Check sheet for the modelled part. Datum: model origin and axes. Units: mm. A direction names the side the tool comes from. Coordinates: 2 decimals unless noted, no trailing zeros. Loops run counter-clockwise (first coordinate to the right, second up) from the corner with the lowest first, then second, coordinate; pieces in that order, holes last. Notation, with made-up numbers: (40.25, 75.5) - (97.25, 75.5) arc R10 cw to (97.25, 81.5) - close; hole circle Ø10 at (48.5, 21.5). An arc over 180 degrees is marked (long way). Use a Markdown table: item, result. Add a question column.
1) Sectioned sample at B-B, the plane y = 0. Enter the section's corners in (x, z), then the cut area to 4 significant figures.
2) Draft check along Y on faces 1 (the flat face through (0, 0, 17)), 2 (the flat face through (0, 2, 10.5)), 3 (the cylindrical face through (-2.17, -9.76, 8.38)). Enter one of: pulls with the +Y half, pulls with the -Y half, needs draft (parallel to the pull), parting line crosses it, or undercut.
3) Go/stop test with flat-tipped pins: P1, Ø1.3, axis at x = 1, y = 1, coming from the -Z side; P2, Ø10, axis at y = 7, z = 13, coming from the +X side; P3, Ø2, axis at y = -6.5, z = 11.5, coming from the +X side; P4, Ø8, axis at y = -3.5, z = 8, coming from the -X side. Record where each tip stops, or that it passes through.
4) Sectioned sample at A-A, the plane x = 0. Enter the section's corners in (y, z).
5) Sectioned sample at D-D, the plane z = 2.25. Enter the section's corners in (x, y), then the cut area to 3 significant figures.
6) Thickness scan on line 1 (Y direction, x = 0, z = 2.1); line 2 (Z direction, x = 5, y = -1.25); line 3 (X direction, y = 6.25, z = 2.5). Record the ranges inside material, lowest first.
7) Sectioned sample at C-C, the plane z = 8. Enter the section's corners in (x, y), then the cut area to 3 significant figures.
8) Tool access check on faces 4 (the flat face through (4, 7, 0)), 5 (the flat face through (0, 0, 3.5)). Record the directions out of +Z, -Z, +X, -X, +Y, -Y that give a thin tool (end or side, any length) a straight path to the whole face; none if there is none.
from build123d import *

# Parameters (mm, degrees)
SKETCH1_R           = 10
BOSS_EXTRUDE1_DEPTH = 17
SKETCH2_R           = 7.5
CUT_EXTRUDE1_DEPTH  = 3.5
CUT_EXTRUDE2_DEPTH  = 7


with BuildPart() as part:
    # Sketch1 → Boss-Extrude1 (new body)
    with BuildSketch(Plane.XY):
        Circle(SKETCH1_R)
    extrude(amount=BOSS_EXTRUDE1_DEPTH)

    # Sketch2 → Cut-Extrude1 (cut)
    with BuildSketch(Plane(origin=(0, 0, 0), x_dir=(-1, 0, 0), z_dir=(0, 0, -1))):
        Circle(SKETCH2_R)
    extrude(amount=-CUT_EXTRUDE1_DEPTH, mode=Mode.SUBTRACT)

    # Sketch4 → Cut-Extrude2 (cut)
    with BuildSketch(Plane(origin=(0, 0, 3.5), x_dir=(-1, 0, 0), z_dir=(0, 0, -1))):
        with BuildLine():
            Line((-3.059411708, 0.5), (3.059411708, 0.5))
            ThreePointArc((3.059411708, 0.5), (0, 3.1), (-3.059411708, 0.5))
        make_face()
        with BuildLine():
            Line((-3.059411708, -0.5), (3.059411708, -0.5))
            ThreePointArc((3.059411708, -0.5), (0, -3.1), (-3.059411708, -0.5))
        make_face()
    extrude(amount=-CUT_EXTRUDE2_DEPTH, mode=Mode.SUBTRACT)


solid = part.part
Solved:
| question | item | result |
|---|---|---|
| 1 | outline | (-10, 0) - (-7.5, 0) - (-7.5, 3.5) - (7.5, 3.5) - (7.5, 0) - (10, 0) - (10, 17) - (-10, 17) - close |
| 1 | area | 287.5 mm2 |
| 2 | face 1 | needs draft |
| 2 | face 2 | undercut |
| 2 | face 3 | parting line crosses it |
| 3 | P1 | stops at z = 3.5 |
| 3 | P2 | stops at x = 9.8 |
| 3 | P3 | stops at x = 8.35 |
| 3 | P4 | stops at x = -10 |
| 4 | outline | (-10, 0) - (-7.5, 0) - (-7.5, 3.5) - (-3.1, 3.5) - (-3.1, 10.5) - (-0.5, 10.5) - (-0.5, 3.5) - (0.5, 3.5) - (0.5, 10.5) - (3.1, 10.5) - (3.1, 3.5) - (7.5, 3.5) - (7.5, 0) - (10, 0) - (10, 17) - (-10, 17) - close |
| 5 | outline | circle Ø20 at (0, 0); hole circle Ø15 at (0, 0) |
| 5 | area | 137 mm2 |
| 6 | line 1 | y = -10 to -7.5, 7.5 to 10 |
| 6 | line 2 | z = 3.5 to 17 |
| 6 | line 3 | x = -7.81 to -4.15, 4.15 to 7.81 |
| 7 | outline | circle Ø20 at (0, 0); hole (-3.06, -0.5) arc R3.1 ccw to (3.06, -0.5) - close; hole (-3.06, 0.5) - (3.06, 0.5) arc R3.1 ccw to start |
| 7 | area | 290 mm2 |
| 8 | face 4 | -Z, +X, -X, +Y, -Y |
| 8 | face 5 | -Z |
